Input: dimensioned drawing with shaded views. Units: mm. Origin: part minimum x, y, z. A direction names the side the tool comes from. Round coordinates to 2 decimals unless told otherwise and drop trailing zeros. Loops run counter-clockwise (first coordinate to the right, second up) from the corner with the lowest first, then second, coordinate; pieces in that order, holes last. Notation, with made-up numbers: M 52,-37 L 91,-37 A22 ccw 91,1 Z; hole C -9.75,74.5 d3. An arc over 180 degrees is marked long. Use one line per item in the form item = value. Start each with the question number.
Q1. Section query B-B, the plane y = 1.7. Output: boundary loops of the cut face in (x, z).
Q2. Section query C-C, the plane z = 2. Output: boundary loops of the cut face in (x, y) (1 decimal).
Q3. Access query for the marked faces 1 and 2. Directions: +Z, -Z, +X, -X, +Y, -Y. A direction counts if a zero-diameter tool reaches every point of the face in a straight line with its end or side. Return the directions, or none.
Q4. First-contact query: P1, Ø0.7, axis at x = 4.5, z = 2, coming from the +Y side. Flat tip, straight axial feed; report the tip coordinate or a pass-through.
Q5. Mould query, pull axis X, two halves, no side actions, for the marked faces 3, 4, 5 and 6. Classes: pulls with the +X half, pulls with the -X half, needs draft (parallel to the pull), parting line crosses it, or undercut.
Q6. Ray query, line 1 along X through (y, z) = (2.2, 2); line 2 along X through (y, z) = (2.4, 6.5); line 3 along X through (y, z) = (0.2, 2.75) (1 decimal). Return the intervals inside material, ascending.
Q7. Section query D-D, the plane x = 5.5. Output: boundary loops of the cut face in (y, z) (1 decimal).
Q8. Section query A-A, the plane x = 4.5. Output: boundary loops of the cut face in (y, z) (1 decimal), and give its area (3 significant figures).
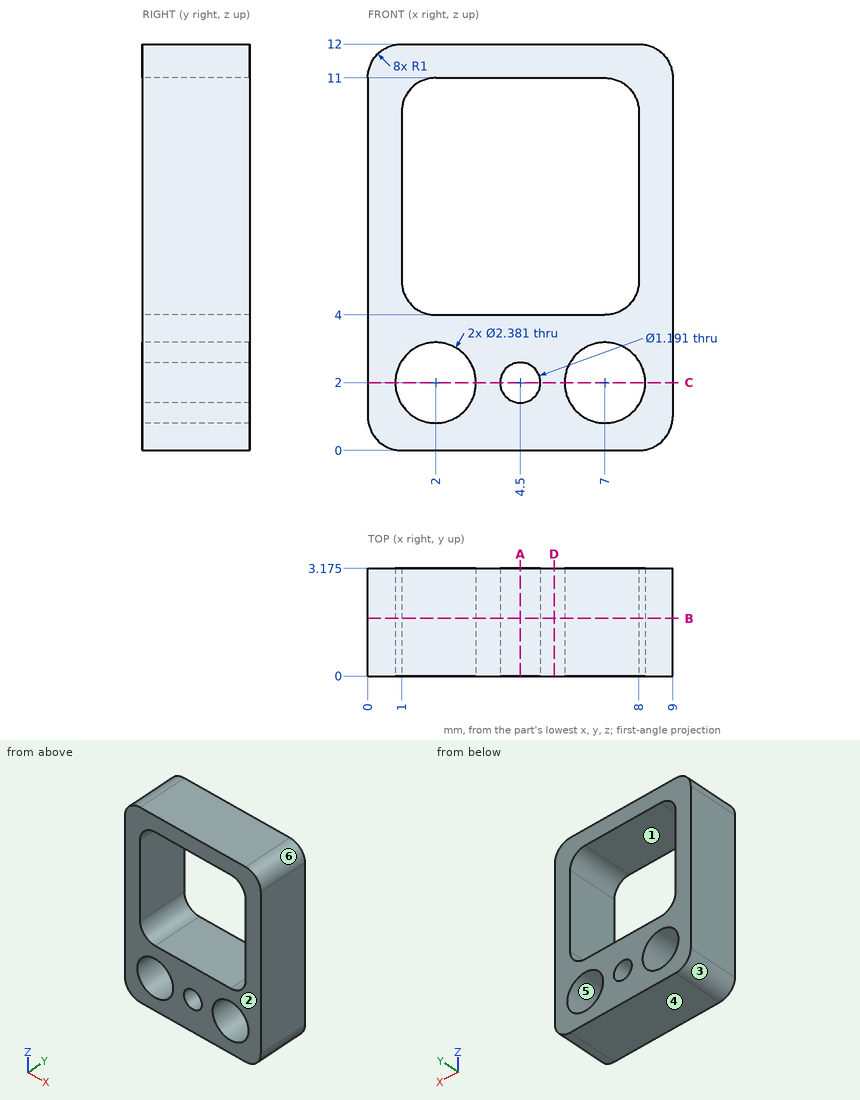
Results found:
q1.outline = M 0,1 A1 ccw 1,0 L 8,0 A1 ccw 9,1 L 9,11 A1 ccw 8,12 L 1,12 A1 ccw 0,11 Z; hole C 2,2 d2.38; hole M 1,5 A1 ccw 2,4 L 7,4 A1 ccw 8,5 L 8,10 A1 ccw 7,11 L 2,11 A1 ccw 1,10 Z; hole C 4.5,2 d1.19; hole C 7,2 d2.38
q2.outline = M 0,0 L 0.8,0 L 0.8,3.2 L 0,3.2 Z; M 3.2,0 L 3.9,0 L 3.9,3.2 L 3.2,3.2 Z; M 5.1,0 L 5.8,0 L 5.8,3.2 L 5.1,3.2 Z; M 8.2,0 L 9,0 L 9,3.2 L 8.2,3.2 Z
q3.face_1 = +Y, -Y
q3.face_2 = +Z, -Z, +X, -X, -Y
q4.P1 = through
q5.face_3 = pulls with the -X half
q5.face_4 = needs draft
q5.face_5 = undercut
q5.face_6 = pulls with the +X half
q6.line_1 = 0 to 0.81, 3.19 to 3.9, 5.1 to 5.81, 8.19 to 9
q6.line_2 = 0 to 1, 8 to 9
q6.line_3 = 0 to 1.1, 2.9 to 6.1, 7.9 to 9
q7.outline = M 0,0 L 3.2,0 L 3.2,4 L 0,4 Z; M 0,11 L 3.2,11 L 3.2,12 L 0,12 Z
q8.outline = M 0,0 L 3.2,0 L 3.2,1.4 L 0,1.4 Z; M 0,2.6 L 3.2,2.6 L 3.2,4 L 0,4 Z; M 0,11 L 3.2,11 L 3.2,12 L 0,12 Z
q8.area = 12.1 mm²
